Read the model definition and answer for the solid it produces. Units are mm, in the model's axes. Face numbers are marked on the shaded views. A direction names the side the tool comes from. Give positions to 0.01 mm unless a question says otherwise; leave off trailing zeros. Write each loop counter-clockwise with the first axis right and the second up, starting at its lowest first coordinate (ties: lowest second). Pieces come first, ordered by that corner, then holes. Notation, with made-up numbers: (30.5, 21) - (57.5, 21) arc R34 ccw to (57.5, 57) - close; hole circle Ø7 at (-36.75, 32). An arc over 180 degrees is marked (long way). Answer as a JSON object with one key per item and string values. Group by question number.
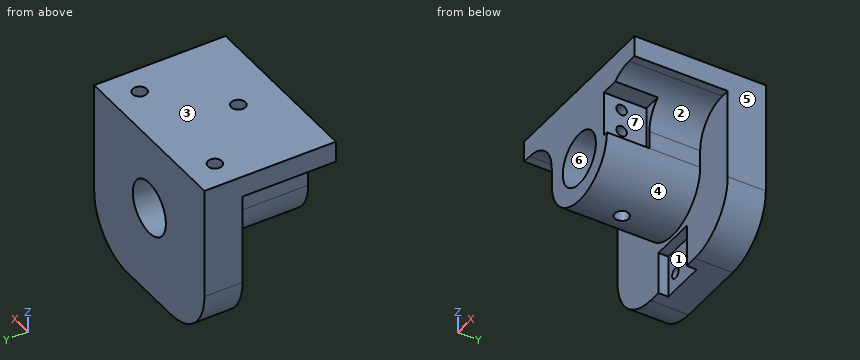
```python
from build123d import *

# Parameters (mm, degrees)
PROFILE_SKETCH1_R                              = 7.5
PROFILE_BOSS_EXTRUDE2_DEPTH                    = 37.25987
FASTENINGHOLESKETCH3_R                         = 2
FASTENINGHOLECUT_EXTRUDE8_DEPTH                = 56.995963358
LM8UUFASTENINGHOLESKETCH5_R                    = 2
LM8UUFASTENINGHOLECUT_EXTRUDE9_DEPTH           = 56.995963425
YAXISMICROSWITCHCUT_EXTRUDE1_DEPTH             = 12.05
MICROSWITCHMOUNTINGHOLESKETCH2_R               = 1.5
YAXISMICROSWITCHMOUNTINGHOLECUT_EXTRUDE2_DEPTH = 3.1
TOPKNOTCHSKETCH2_W                             = 50
TOPKNOTCHSKETCH2_H                             = 27.5
TOPKNOTCHCUT_EXTRUDE1_DEPTH                    = 10.8
TOPSHELFSKETCH3_W                              = 50
TOPSHELFSKETCH3_H                              = 10.8
TOPSHELFBOSS_EXTRUDE1_DEPTH                    = 40.75
TOPSHELFLM8UUHOLESKETCH_R                      = 7.5
TOPSHELFLM8UUCUT_EXTRUDE2_DEPTH                = 52.733552168
XAXISMICROSWITCHSKETCH7_W                      = 12.85
XAXISMICROSWITCHSKETCH7_H                      = 12.05
XAXISMICROSWITCHCUT_EXTRUDE5_DEPTH             = 2.8
XAXISMICROSWITCHMOUNTINGHOLESKETCH8_R          = 1.5
XAXISMICROSWITCHMOUNTINGHOLECUT_EXTRUDE6_DEPTH = 3.1
FILLET3_R                                      = 15
FILLET4_R                                      = 15


with BuildPart() as part:
    # Profile-Sketch1 → Profile-Boss-Extrude2 (new body)
    with BuildSketch(Plane(origin=(0, 0, 0), x_dir=(1, 0, 0), z_dir=(0, 1, 0))):
        with BuildLine():
            Line((-25, -21), (25, -21))
            Line((25, -21), (25, -15))
            Line((25, -15), (22.5, -15))
            ThreePointArc((22.5, -15), (15.428932188, -12.071067812), (12.5, -5))
            Line((12.5, -5), (12.5, 0))
            ThreePointArc((12.5, 0), (0, 12.5), (-12.5, 0))
            Line((-12.5, 0), (-12.5, -5))
            ThreePointArc((-12.5, -5), (-15.428932188, -12.071067812), (-22.5, -15))
            Line((-22.5, -15), (-25, -15))
            Line((-25, -15), (-25, -21))
        make_face()
        with Locations(Location((0, 0, 0), (0, 0, 270))):
            Circle(PROFILE_SKETCH1_R, mode=Mode.SUBTRACT)
    extrude(amount=PROFILE_BOSS_EXTRUDE2_DEPTH)

    # FasteningHoleSketch3 → FasteningHoleCut-Extrude8 (cut, through all)
    with BuildSketch(Plane.XY.offset(21)):
        with Locations((-17.0625, 29.32237)):
            Circle(FASTENINGHOLESKETCH3_R)
        with Locations((17.0625, 29.32237)):
            Circle(FASTENINGHOLESKETCH3_R)
    extrude(amount=-FASTENINGHOLECUT_EXTRUDE8_DEPTH, mode=Mode.SUBTRACT)

    # LM8UUFasteningHoleSketch5 → LM8UUFasteningHoleCut-Extrude9 (cut, through all)
    with BuildSketch(Plane.XY.offset(21)):
        with Locations((0, 12)):
            Circle(LM8UUFASTENINGHOLESKETCH5_R)
    extrude(amount=-LM8UUFASTENINGHOLECUT_EXTRUDE9_DEPTH, mode=Mode.SUBTRACT)

    # Sketch1 → YAxisMicroSwitchCut-Extrude1 (cut)
    with BuildSketch(Plane.XZ):
        Polygon((13.9, 12.85), (16.363847734, 12.85), (13.9, 10.102940329), (13.9, 0), (11.1, 0), (11.1, 12.85), align=None)
    extrude(amount=-YAXISMICROSWITCHCUT_EXTRUDE1_DEPTH, mode=Mode.SUBTRACT)

    # MicroSwitchMountingHoleSketch2 → YAxisMicroSwitchMountingHoleCut-Extrude2 (cut)
    with BuildSketch(Plane(origin=(11.1, 0, 0), x_dir=(0, 0, -1), z_dir=(1, 0, 0))):
        with Locations((-9.6, 5.05)):
            Circle(MICROSWITCHMOUNTINGHOLESKETCH2_R)
        with Locations((-3.25, 5.05)):
            Circle(MICROSWITCHMOUNTINGHOLESKETCH2_R)
    extrude(amount=-YAXISMICROSWITCHMOUNTINGHOLECUT_EXTRUDE2_DEPTH, mode=Mode.SUBTRACT)

    # TopKnotchSketch2 → TopKnotchCut-Extrude1 (cut)
    with BuildSketch(Plane(origin=(0, 37.25987, 0), x_dir=(1, 0, 0), z_dir=(0, 1, 0))):
        with Locations((0, -1.25)):
            Rectangle(TOPKNOTCHSKETCH2_W, TOPKNOTCHSKETCH2_H)
    extrude(amount=-TOPKNOTCHCUT_EXTRUDE1_DEPTH, mode=Mode.SUBTRACT)

    # TopShelfSketch3 → TopShelfBoss-Extrude1 (add)
    with BuildSketch(Plane(origin=(0, 0, 15), x_dir=(-1, 0, 0), z_dir=(0, 0, -1))):
        with Locations((0, 31.85987)):
            Rectangle(TOPSHELFSKETCH3_W, TOPSHELFSKETCH3_H)
    extrude(amount=TOPSHELFBOSS_EXTRUDE1_DEPTH)

    # TopShelfLM8UUHoleSketch → TopShelfLM8UUCut-Extrude2 (cut, through all)
    with BuildSketch(Plane(origin=(0, 37.25987, 0), x_dir=(1, 0, 0), z_dir=(0, 1, 0))):
        with Locations(Location((0, 0, 0), (0, 0, 270))):
            Circle(TOPSHELFLM8UUHOLESKETCH_R)
    extrude(amount=-TOPSHELFLM8UUCUT_EXTRUDE2_DEPTH, mode=Mode.SUBTRACT)

    # XAxisMicroSwitchSketch7 → XAxisMicroSwitchCut-Extrude5 (cut)
    with BuildSketch(Plane.XZ.offset(-26.45987)):
        with Locations((0, -19.725)):
            Rectangle(XAXISMICROSWITCHSKETCH7_W, XAXISMICROSWITCHSKETCH7_H)
    extrude(amount=-XAXISMICROSWITCHCUT_EXTRUDE5_DEPTH, mode=Mode.SUBTRACT)

    # XAxisMicroSwitchMountingHoleSketch8 → XAxisMicroSwitchMountingHoleCut-Extrude6 (cut)
    with BuildSketch(Plane.XZ.offset(-29.25987)):
        with Locations(Location((-3.175, -20.7, 0), (0, 0, 270))):
            Circle(XAXISMICROSWITCHMOUNTINGHOLESKETCH8_R)
        with Locations(Location((3.175, -20.7, 0), (0, 0, 270))):
            Circle(XAXISMICROSWITCHMOUNTINGHOLESKETCH8_R)
    extrude(amount=-XAXISMICROSWITCHMOUNTINGHOLECUT_EXTRUDE6_DEPTH, mode=Mode.SUBTRACT)

    # Fillet3
    fillet3_edges = [part.edges().sort_by_distance(p)[0] for p in [
        (25, 31.85987, -25.75),
    ]]
    fillet(fillet3_edges, radius=FILLET3_R)

    # Fillet4
    fillet4_edges = [part.edges().sort_by_distance(p)[0] for p in [
        (-25, 31.85987, -25.75),
    ]]
    fillet(fillet4_edges, radius=FILLET4_R)


solid = part.part
```
1) Find the intervals of material crossed by line 1 (Z direction, x = 10, y = 5); line 2 (Z direction, x = 0, y = 30); line 3 (X direction, y = 30, z = 0), in increasing order. Write a range as [from, to].
2) Flat-ended cylindrical pins translate along their axes: pin 1 Ø2.5 at (x, y) = (17.06, 29.32) entering from +Z; pin 2 Ø3 at (x, y) = (-17.06, 29.32) entering from -Z; pin 3 Ø1 at (y, z) = (20, 12.5) entering from -X; pin 4 Ø10 at (y, z) = (5, -19) entering from -X. Find the tip coordinate at first contact, or state that the pin passes through.
3) Find section B-B, the plane x = 0. Write down the section's boundary in (y, z), and give its area (3 significant figures).
4) Find section A-A, the plane y = 24.5. Write down the section's boundary in (x, z).
5) For a pull along Z with two mould halves and no side action, classify the marked faces 4, 5, 6 and 7 as released by +Z, released by -Z, zero draft, split by the parting line, or undercut.
6) Which of the six approach directions +Z, -Z, +X, -X, +Y, -Y give full straight-line access (tool end or side, diameter ignored) to the marked faces 1, 2 and 3?
7) Find section C-C, the plane z = -1. Write down the section's boundary in (x, y), and give its area (3 significant figures).
8) Find section D-D, the plane z = 9.6. Write down the section's boundary in (x, y), and give its area (3 significant figures).
Values follow:
{
 "1": {"line 1": "z = [-7.5, 1.75], [4.75, 8.1], [11.1, 21]", "line 2": "z = [-25.75, -7.5], [7.5, 21]", "line 3": "x = [-25, -7.5], [7.5, 25]"},
 "2": {"pin 1": "stops at z = 15", "pin 2": "stops at z = -24.68", "pin 3": "stops at x = -16.5", "pin 4": "passes through"},
 "3": {"outline": "(0, -12.5) - (10, -12.5) - (10, -7.5) - (0, -7.5) - close; (0, 7.5) - (10, 7.5) - (10, 21) - (0, 21) - close; (14, -12.5) - (26.46, -12.5) - (26.46, -13.7) - (29.26, -13.7) - (29.26, -25.75) - (37.26, -25.75) - (37.26, -7.5) - (14, -7.5) - close; (14, 7.5) - (37.26, 7.5) - (37.26, 21) - (14, 21) - close", "area": "725 mm2"},
 "4": {"outline": "(-25, 15) - (-22.5, 15) arc R10 cw to (-12.5, 5) - (-12.5, 0) arc R12.5 ccw to (12.5, 0) - (12.5, 5) arc R10 cw to (22.5, 15) - (25, 15) - (25, 21) - (-25, 21) - close; hole circle Ø15 at (0, 0)"},
 "5": {"face 4": "released by -Z", "face 5": "zero draft", "face 6": "undercut", "face 7": "undercut"},
 "6": {"face 1": "-Z, -Y", "face 2": "-Z, +X, -Y", "face 3": "+Z, +X, -X, +Y, -Y"},
 "7": {"outline": "(-25, 26.46) - (-12.46, 26.46) - (-12.46, 0) - (-7.43, 0) - (-7.43, 37.26) - (-25, 37.26) - close; (7.43, 0) - (12.46, 0) - (12.46, 26.46) - (25, 26.46) - (25, 37.26) - (7.43, 37.26) - close", "area": "645 mm2"},
 "8": {"outline": "(-25, 26.46) - (-13.62, 26.46) - (-13.62, 0) - (11.1, 0) - (11.1, 3.55) - (8, 3.55) - (8, 6.55) - (11.1, 6.55) - (11.1, 12.05) - (13.62, 12.05) - (13.62, 26.46) - (25, 26.46) - (25, 37.26) - (-25, 37.26) - close; hole circle Ø4 at (0, 12)", "area": "1,210 mm2"}
}
